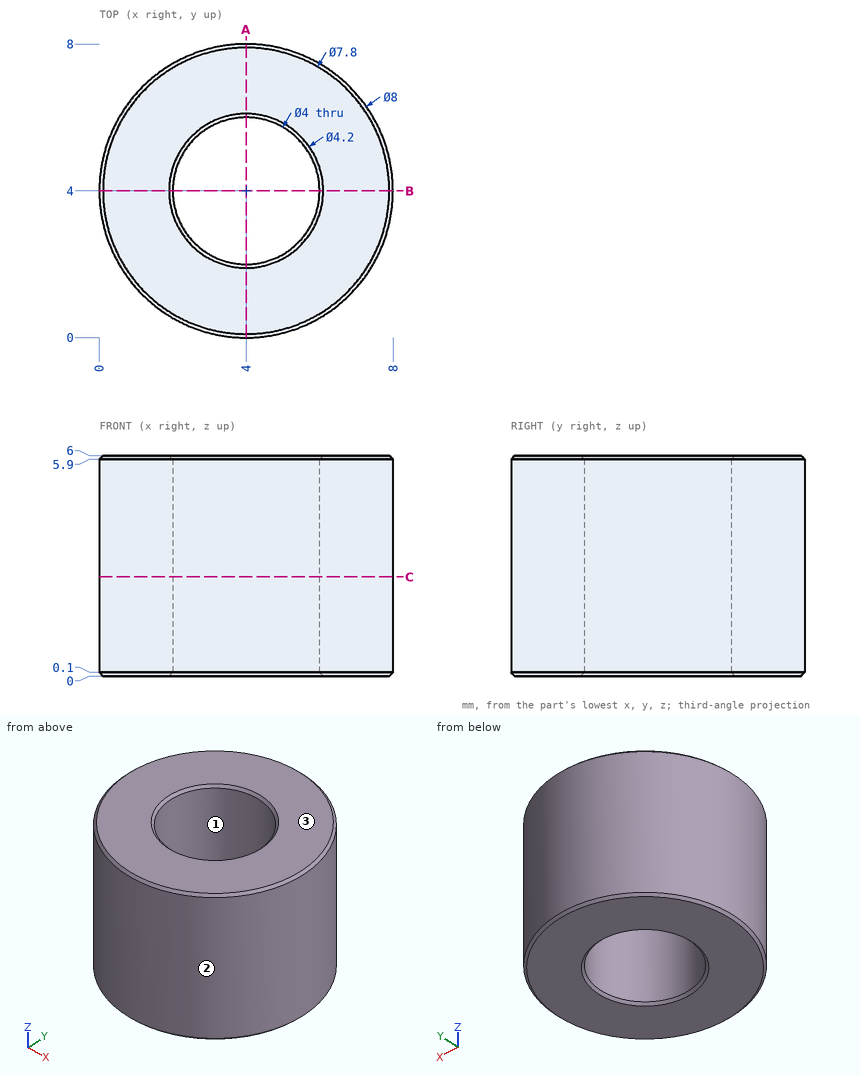
The figure shows three views and two pictorial views of one solid part (mm, origin at its lowest corner). Answer the questions. Give positions to 0.01 mm unless a question says otherwise; leave off trailing zeros. Loops run counter-clockwise (first coordinate to the right, second up) from the corner with the lowest first, then second, coordinate; pieces in that order, holes last. Notation, with made-up numbers: (33.25, -1.5) -> (76.25, -1.5) arc R22 ccw to (76.25, 9.5) -> close; hole circle Ø8 at (-34.5, -36.75). An arc over 180 degrees is marked (long way). Use a Markdown table: item, result. Add a question column.
1. Find the intervals of material crossed by probe 1 along Y at (x, z) = (4, 2.45); probe 2 along X at (y, z) = (3.5, 1.25); probe 3 along Y at (x, z) = (2.75, 1.1), in increasing order.
2. Section A-A on x = 4 is taken. Determine the outline of the cut face in (y, z), and give its area (3 significant figures).
3. Section C-C on z = 2.7 is taken. Determine the outline of the cut face in (x, y), and give its area (3 significant figures).
4. A flat-ended cylindrical pin translates along its axis: pin 1 Ø2 at (x, z) = (6, 1) entering from +Y. Find the tip coordinate at first contact, or state that the pin passes through.
5. Determine the mould class of the marked faces 1, 2 and 3 for opening direction Y: released by +Y, released by -Y, zero draft, split by the parting line, or undercut.
Results below:
| question | item | result |
|---|---|---|
| 1 | probe 1 | y = 0 to 2, 6 to 8 |
| 1 | probe 2 | x = 0.03 to 2.06, 5.94 to 7.97 |
| 1 | probe 3 | y = 0.2 to 2.44, 5.56 to 7.8 |
| 2 | outline | (0, 0.1) -> (0.1, 0) -> (1.9, 0) -> (2, 0.1) -> (2, 5.9) -> (1.9, 6) -> (0.1, 6) -> (0, 5.9) -> close; (6, 0.1) -> (6.1, 0) -> (7.9, 0) -> (8, 0.1) -> (8, 5.9) -> (7.9, 6) -> (6.1, 6) -> (6, 5.9) -> close |
| 2 | area | 24.0 mm^2 |
| 3 | outline | circle Ø8 at (4, 4); hole circle Ø4 at (4, 4) |
| 3 | area | 37.7 mm^2 |
| 4 | pin 1 | stops at y = 7.87 |
| 5 | face 1 | undercut |
| 5 | face 2 | split by the parting line |
| 5 | face 3 | zero draft |
